Geometry: final body of the model. Coordinates: model frame, mm. Face numbers are marked on the shaded views. A direction names the side the tool comes from. Coordinates: 2 decimals unless noted, no trailing zeros. Write each loop counter-clockwise with the first axis right and the second up, starting at its lowest first coordinate (ties: lowest second). Pieces come first, ordered by that corner, then holes. Notation, with made-up numbers: (81.5, 31) - (127.5, 31) arc R9 ccw to (127.5, 37) - close; hole circle Ø4 at (33.5, -4). An arc over 180 degrees is marked (long way). Put each result on its own line as item: value.
Autodesk Inventor part; units mm, degrees
ref_plane "MidPlane" through (0, -13.6061, 0) normal (-1, 0, 0) x (0, 0, -1)
ref_plane "YZ Plane" through (0, 0, 0) normal (1, 0, 0) x (0, 1, 0)
ref_plane "XZ Plane" through (0, 0, 0) normal (0, 1, 0) x (-1, 0, 0)
sketch "Base" plane through (0, 0, 0) normal (0, 0, 1) x (1, 0, 0)
  line L0 (-7.5, 5.4092) -> (-3, 10.5)
  line L1 (-3, -6) -> (-3, -10)
  line L2 (-7.5, 5.4092) -> (-3, -6)
  line L3 (0, 10.5) -> (0, -10) construction
  line L4 (7.5, 5.4092) -> (3, 10.5)
  line L5 (3, -6) -> (3, -10)
  line L6 (7.5, 5.4092) -> (3, -6)
  circle A0 centre (0, 0) radius 1
  line L7 (0.5297, 6.5) -> (3.417, 3.2336) construction
  line L8 (2.5405, 8) -> (4.8181, 5.4233) construction
  circle A1 centre (0.5297, 6.5) radius 0.75
  circle A2 centre (2.5405, 8) radius 0.75
  circle A3 centre (3.417, 3.2336) radius 0.75
  circle A4 centre (4.8181, 5.4233) radius 0.75
  line L9 (-3, 10.5) -> (3, 10.5)
  line L10 (-3, -10) -> (3, -10)
  line L11 (3.1024, 8.4967) -> (5.3801, 5.92)
  line L12 (1.9786, 7.5033) -> (4.2562, 4.9266)
  line L13 (1.0917, 6.9967) -> (3.9789, 3.7303)
  line L14 (-0.0322, 6.0033) -> (2.8551, 2.7369)
  dimension "d13" = 2
  dimension "d14" = 1.5
  dimension "d17" = 2
  dimension "d18" = 2.5
  dimension "d20" = 6
  dimension "d23" = 117
  dimension "d24" = 6
  dimension "d25" = 15
  dimension "d26" = 4
  dimension "d28" = 2.5
  dimension "d29" = 3
  dimension "d30" = 2.5
  dimension "d31" = 4
  dimension "d32" = 16.5
  dimension "d56" = 10
extrude "BaseFeature" add sketch "Base" along normal blind 6.5
ref_plane "MidPlane" through (0, -13.6061, 0) normal (-1, 0, 0) x (0, 0, -1)
sketch "SideProfile" plane through (0, -13.6061, 0) normal (-1, 0, 0) x (0, 0, -1)
  line L0 (0, -24.1061) -> (-6.5, -24.1061)
  line L1 (-6.5, -7.6061) -> (-3, -24.1061)
  line L2 (-3, -24.1061) -> (0, -24.1061)
  line L3 (0, -24.1061) -> (0, -7.6061)
  line L4 (-6.5, -3.6061) -> (-6.5, -7.6061)
  line L5 (-6.5, -3.6061) -> (0, -3.6061)
  line L6 (0, -3.6061) -> (0, -7.6061)
  dimension "d37" = 3
extrude "SideProfileFeature" cut sketch "SideProfile" along normal through all both and the other way through all keep common part
fillet "BaseFilletsFeature" radius 1 8 edges at (-3, 10.5, 1.5) (-7.5, 5.4092, 2.0399) (-3, -6, 3.25) (-3, -10, 3.25) (3, -10, 3.25) (3, -6, 3.25) (7.5, 5.4092, 2.0399) (3, 10.5, 1.5)
sketch "FrontHole" plane through (-2, -10, 6.5) normal (0, -1, 0) x (1, 0, 0)
  circle A0 centre (2, -3.25) radius 1.25
  line L0 (0, -6.5) -> (4, -6.5)
  line L1 (0, 0) -> (4, 0)
  line L2 (4, 0) -> (4, -6.5)
  line L3 (0, -6.5) -> (0, 0)
  dimension "d41" = 2.5
  dimension "d42" = 6.5
  dimension "d43" = 4
  dimension "d44" = 3.25
  dimension "d45" = 2
hole "FrontHoleFeature" at (0, -10, 3.25) direction (0, 1, 0) diameter 2 depth 6 tip angle 118
equation "\"d44\" = 0.5 * d42"
equation "\"d45\" = 0.5 * d43"
properties part number "ForearmPistonConnector"
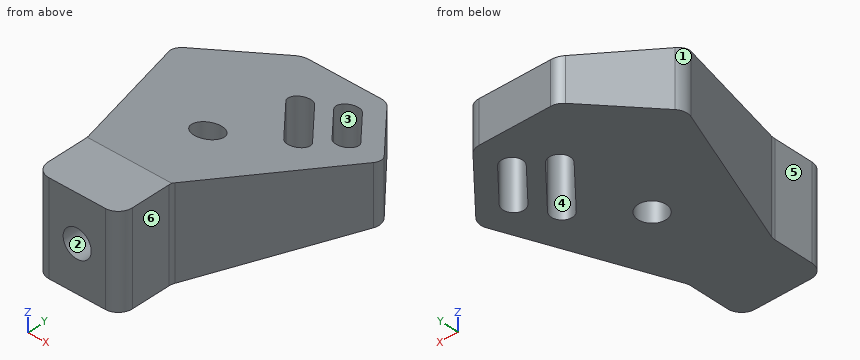
1. Set-up query: the marked faces 4, 5 and 6. Return all of +Z, -Z, +X, -X, +Y, -Y with unobstructed straight access to the full face (end or side cutting, diameter ignored); none if empty.
Answer below:
face 4: +Z, -Z
face 5: +Z, -Z, -X, -Y
face 6: +Z, -Z, +X, -Y
2. Pin query (flat end, axial travel): pin 1 Ø4 at (x, y) = (2, -6) entering from -Z; pin 2 Ø3 at (y, z) = (-7.5, 1) entering from -X; pin 3 Ø3 at (x, y) = (0, 0) entering from +Z; pin 4 Ø1.4 at (y, z) = (-7.5, 2.5) entering from +X. Return the tip coordinate at first contact, or that it passes through.
Answer below:
pin 1: stops at z = 0
pin 2: stops at x = -3.02
pin 3: stops at z = 5.55
pin 4: stops at x = 3
3. Mould query, pull axis Y, two halves, no side actions, for the marked faces 1, 2 and 3. Classes: +Y half, -Y half, draft (parallel to the pull), parting line (faces both ways), or undercut.
Answer below:
face 1: parting line
face 2: draft
face 3: undercut
4. Section query C-C (z = 1.25). Return loops of the section in (x, y).
Answer below:
outline: (-7.28, 4.84) - (-3.07, -5.82) arc R1 cw to (-3, -6.19) - (-3, -9) arc R1 ccw to (-2, -10) - (2, -10) arc R1 ccw to (3, -9) - (3, -6.19) arc R1 cw to (3.07, -5.82) - (7.28, 4.84) arc R1 ccw to (7.09, 5.87) - (3.3, 10.16) arc R1 ccw to (2.55, 10.5) - (-2.55, 10.5) arc R1 ccw to (-3.3, 10.16) - (-7.09, 5.87) arc R1 ccw to start; hole circle Ø2 at (0, 0); hole (-0.03, 6) - (2.86, 2.74) arc R0.75 ccw to (3.98, 3.73) - (1.09, 7) arc R0.75 ccw to start; hole (1.98, 7.5) - (4.26, 4.93) arc R0.75 ccw to (5.38, 5.92) - (3.1, 8.5) arc R0.75 ccw to start
5. Section query B-B (y = 8). Return loops of the section in (x, z), then the cut area to 3 significant figures.
Answer below:
outline: (-5.21, 0) - (1.79, 0) - (1.79, 3.53) - (-5.21, 3.53) - close; (3.54, 0) - (5.21, 0) - (5.21, 3.53) - (3.54, 3.53) - close
area: 30.6 mm²
6. Section query A-A (y = -8.5). Return loops of the section in (x, z).
Answer below:
outline: (-3, 0) - (3, 0) - (3, 6.5) - (-3, 6.5) - close; hole circle Ø2 at (0, 3.25)
7. Section query D-D (z = 6). Return loops of the section in (x, y), then the cut area to 3 significant figures.
Answer below:
outline: (-3.93, -3.64) - (-3.07, -5.82) arc R1 cw to (-3, -6.19) - (-3, -9) arc R1 ccw to (-2, -10) - (2, -10) arc R1 ccw to (3, -9) - (3, -6.19) arc R1 cw to (3.07, -5.82) - (3.93, -3.64) - close
area: 39.9 mm²
8. Ray query, probe 1 along Z at (x, y) = (0, -7.25); probe 2 along X at (y, z) = (-8.2, 3.25); probe 3 along Y at (x, z) = (2.75, 2). Return the intervals inside material, ascending. Write a range as from..to.
Answer below:
probe 1: z = 0..2.25, 4.25..6.5
probe 2: x = -3..-1, 1..3
probe 3: y = -9.66..2.86, 5.12..6.63, 8.72..10.48
